```python
from build123d import *

# Parameters (mm, degrees)
BOSS_EXTRUDE2_DEPTH             = 3
BOSS_EXTRUDE3_DEPTH             = 25
SKETCH11_R                      = 3.5
BOSS_EXTRUDE5_DEPTH             = 7
BOSS_EXTRUDE5_DIRECTION_2_REACH = 85.256


with BuildPart() as part:
    # Sketch1 → Boss-Extrude2 (new body)
    with BuildSketch(Plane(origin=(0, 0, 0), x_dir=(1, 0, 0), z_dir=(0, 1, 0))):
        with BuildLine():
            Line((0, 0), (0, -70))
            Line((0, -70), (70, -70))
            Line((70, -70), (70, -20))
            ThreePointArc((70, -20), (36.231761047, -5.688836334), (0, 0))
        make_face()
    extrude(amount=BOSS_EXTRUDE2_DEPTH)

    # Sketch3 → Boss-Extrude3 (add)
    with BuildSketch(Plane(origin=(0, 3, 0), x_dir=(1, 0, 0), z_dir=(0, 1, 0))):
        with BuildLine():
            Line((70, -70), (70, -20))
            ThreePointArc((70, -20), (36.231761047, -5.688836334), (0, 0))
            Line((0, 0), (0, -70))
            Line((0, -70), (70, -70))
        make_face()
        with BuildLine():
            Line((3, -3.133993062), (3, -67))
            Line((3, -67), (67, -67))
            Line((67, -67), (67, -21.744121307))
            ThreePointArc((67, -21.744121307), (36.068657655, -8.763956776), (3, -3.133993062))
        make_face(mode=Mode.SUBTRACT)
    extrude(amount=BOSS_EXTRUDE3_DEPTH)

    # Sketch11 → Boss-Extrude5 (add)
    with BuildSketch(Plane(origin=(61.178699811, 14, 15.293872991), x_dir=(-0.8974903699241337, 0, -0.4410340529862085), z_dir=(0.4410340529862085, 0, -0.8974903699241337))):
        with Locations((25.829909239, 0)):
            Circle(SKETCH11_R)
    extrude(amount=BOSS_EXTRUDE5_DEPTH)

    # Sketch11 → Boss-Extrude5 direction 2 (add, up to next)
    with BuildSketch(Plane(origin=(61.178699811, 14, 15.293872991), x_dir=(-0.8974903699241337, 0, -0.4410340529862085), z_dir=(0.4410340529862085, 0, -0.8974903699241337)), mode=Mode.PRIVATE) as boss_extrude5_direction_2_sk1:
        with Locations((25.829909239, 0)):
            Circle(SKETCH11_R)
    boss_extrude5_direction_2_tool1 = extrude(boss_extrude5_direction_2_sk1.sketch, amount=-BOSS_EXTRUDE5_DIRECTION_2_REACH, mode=Mode.PRIVATE) - part.part
    add(boss_extrude5_direction_2_tool1.solids().sort_by_distance((37.996605, 14, 3.902003))[0])


solid = part.part
```
For this review, take the finished solid that the model builds, in its own axes (mm). A direction names the side the tool comes from. Round coordinates to 2 decimals unless told otherwise and drop trailing zeros. Write each loop counter-clockwise with the first axis right and the second up, starting at its lowest first coordinate (ties: lowest second). Pieces come first, ordered by that corner, then holes. Notation, with made-up numbers: M -37.5,-35 L -0.5,-35 A10 cw -0.5,-24 Z; hole C 26.5,-13 d1. An arc over 180 degrees is marked long. One line per item, written item: value. Start each with the question number.
(1) The part is to be moulded in two halves that separate along X. For faces 1 (the flat face through (41.128, 14.049, -2.359)), 2 (the flat face through (0, 14, 35)), 3 (the flat face through (67, 15, 45)), 4 (the flat face through (35, 0, 35)), say which applies: released by +X, released by -X, zero draft, split by the parting line, or undercut.
(2) Machinability: for faces 5 (the flat face through (35, 14, 70)), 6 (the flat face through (3, 15, 35)), which of the approach directions +Z, -Z, +X, -X, +Y, -Y give a long, thin tool a straight path to every point of the face, cutting with its end or side? Answer none if there is none.
(3) Insertion check: pin 1 (6 mm diameter, centred on x = 48, y = 16.5, fed in from -Z); pin 2 (1 mm diameter, centred on x = 21, z = 55, fed in from +Y); pin 3 (6 mm diameter, centred on x = 50, y = 11.5, fed in from -Z). Each pin has a flat end and moves straight along its axis. Give the tip position at first contact, or say it passes through.
(4) We need section B-B (z = 35). Give the boundary of the cut face in (x, y).
(5) Wall thickness on line 1 (X direction, y = 20.75, z = 36.5); line 2 (Z direction, x = 43.5, y = 14.5); line 3 (X direction, y = 13, z = 17.5): over which ranges is each line inside the solid? List them lowest first.
(6) We need section C-C (x = 28). Give the boundary of the cut face in (y, z), and give its area (3 significant figures).
(7) We need section A-A (y = 26). Give the boundary of the cut face in (x, z).
Result:
1. face 1: released by +X
1. face 2: released by -X
1. face 3: undercut
1. face 4: zero draft
2. face 5: +Z, +X, -X, +Y, -Y
2. face 6: +Y
3. pin 1: z = 8.49
3. pin 2: y = 3
3. pin 3: z = 9.21
4. outline: M 0,0 L 70,0 L 70,28 L 67,28 L 67,3 L 3,3 L 3,28 L 0,28 Z
5. line 1: 0 to 3, 67 to 70
5. line 2: -1.19 to 0.56, 7.97 to 11.14, 67 to 70
5. line 3: 0 to 3, 58.86 to 65.49
6. outline: M 0,3.59 L 28,3.59 L 28,6.66 L 3,6.66 L 3,67 L 28,67 L 28,70 L 0,70 Z
6. area: 351 mm²
7. outline: M 0,0 A150 ccw 70,20 L 70,70 L 0,70 Z; hole M 3,3.13 A147 ccw 67,21.74 L 67,67 L 3,67 Z
